from build123d import *

# Parameters (mm, degrees)
SKETCH106_W     = 20
SKETCH106_H     = 35
PAD054_DEPTH    = 10
PAD055_DEPTH    = 10
SKETCH107_R     = 3.9
POCKET042_DEPTH = 35
SKETCH108_R     = 1.5
POCKET043_DEPTH = 10
SKETCH109_R     = 2.5
PAD056_DEPTH    = 5
SKETCH110_R     = 2.5
PAD057_DEPTH    = 5


with BuildPart() as part:
    # Sketch106 → Pad054 (new body, symmetric)
    with BuildSketch(Plane.YZ):
        with Locations((0, -17.5)):
            Rectangle(SKETCH106_W, SKETCH106_H)
    extrude(amount=PAD054_DEPTH, both=True)

    # Sketch106 → Pad055 (join)
    with BuildSketch(Plane.YZ):
        with Locations((0, -17.5)):
            Rectangle(SKETCH106_W, SKETCH106_H)
    extrude(amount=PAD055_DEPTH)

    # Sketch107 (on Face1 of Pad055) → Pocket042 (cut)
    with BuildSketch(Plane.YX.offset(35)):
        Circle(SKETCH107_R)
    extrude(amount=-POCKET042_DEPTH, mode=Mode.SUBTRACT)

    # Sketch108 (on Face9 of Pocket042) → Pocket043 (cut)
    with BuildSketch(Plane.YZ.offset(10)):
        with Locations((0, -7)):
            Circle(SKETCH108_R)
    extrude(amount=-POCKET043_DEPTH, mode=Mode.SUBTRACT)

    # Sketch109 (on Face8 of Pocket043) → Pad056 (join)
    with BuildSketch(Plane.ZX.offset(10)):
        with Locations((-30, 0)):
            Circle(SKETCH109_R)
    extrude(amount=PAD056_DEPTH)

    # Sketch110 (on Face11 of Pad056) → Pad057 (join)
    with BuildSketch(Plane(origin=(0, -10, 0), x_dir=(0, 0, -1), z_dir=(0, -1, 0))):
        with Locations((30, 0)):
            Circle(SKETCH110_R)
    extrude(amount=PAD057_DEPTH)


solid = part.part
Geometry check sheet. Reference: the model listing, model coordinates, mm. A direction names the side the tool comes from. Give positions to 0.01 mm unless a question says otherwise; leave off trailing zeros. Order: outer loops, then holes, each group sorted by start corner. A loop starts at its lowest first (then second) coordinate and runs counter-clockwise, first axis right, second up.
1) Cross-section at B-B (x = 0). Record the boundary of the cut face in (y, z), then the cut area to 3 significant figures.
Results are:
outline: (-15, -32.5) - (-10, -32.5) - (-10, -35) - (-3.9, -35) - (-3.9, 0) - (-10, 0) - (-10, -27.5) - (-15, -27.5) - close; (3.9, -35) - (10, -35) - (10, -32.5) - (15, -32.5) - (15, -27.5) - (10, -27.5) - (10, 0) - (3.9, 0) - close
area: 477 mm2
2) Tool access check on faces 1 (the cylindrical face through (0.1, 12.5, -32.5)), 2 (the flat face through (0, -15, -30)). Record the directions out of +Z, -Z, +X, -X, +Y, -Y that give a thin tool (end or side, any length) a straight path to the whole face; none if there is none.
Results are:
face 1: +Y
face 2: +Z, -Z, +X, -X, -Y
3) Cross-section at A-A (y = 0). Record the boundary of the cut face in (x, z), then the cut area to 3 significant figures.
Results are:
outline: (-10, -35) - (-3.9, -35) - (-3.9, 0) - (-10, 0) - close; (3.9, -35) - (10, -35) - (10, -8.5) - (3.9, -8.5) - close; (3.9, -5.5) - (10, -5.5) - (10, 0) - (3.9, 0) - close
area: 409 mm2
4) Draft check along Z on faces 3 (the cylindrical face through (6.845, -0.325, -8.464)), 4 (the flat face through (0, 10, -18)), 5 (the cylindrical face through (0.1, -12.5, -27.5)). Enter one of: released by +Z, released by -Z, zero draft, split by the parting line, or undercut.
Results are:
face 3: undercut
face 4: zero draft
face 5: split by the parting line
5) Material ranges on probe 1 along Z at (x, y) = (7.5, 0); probe 2 along Y at (x, z) = (5, -7); probe 3 along X at (y, z) = (0, -11.5), recorded low to high.
Results are:
probe 1: z = -35 to -8.5, -5.5 to 0
probe 2: y = -10 to -1.5, 1.5 to 10
probe 3: x = -10 to -3.9, 3.9 to 10
6) Cross-section at D-D (z = -7). Record the boundary of the cut face in (x, y).
Results are:
outline: (-10, -10) - (10, -10) - (10, -1.5) - (3.6, -1.5) arc R3.9 cw (long way) to (3.6, 1.5) - (10, 1.5) - (10, 10) - (-10, 10) - close
7) Cross-section at C-C (z = -30). Record the boundary of the cut face in (x, y).
Results are:
outline: (-10, -10) - (-2.5, -10) - (-2.5, -15) - (2.5, -15) - (2.5, -10) - (10, -10) - (10, 10) - (2.5, 10) - (2.5, 15) - (-2.5, 15) - (-2.5, 10) - (-10, 10) - close; hole circle Ø7.8 at (0, 0)
8) Gauge pin test, flat ends, axial feed: pin 1 (3 mm diameter, centred on x = -2, z = -20, fed in from -Y); pin 2 (8 mm diameter, centred on x = 3.5, z = -15, fed in from +Y); pin 3 (2.5 mm diameter, centred on y = 0, z = -7, fed in from +X). Record the tip position at first contact, or that the pin passes through.
Results are:
pin 1: stops at y = -10
pin 2: stops at y = 10
pin 3: stops at x = -3.69
